from build123d import *

# Parameters (mm, degrees)
SKETCH_1_R               = 2.5
EXTRUDE_1_DEPTH          = 6
SKETCH_2_W               = 4
SKETCH_2_H               = 5
EXTRUDE_2_DEPTH          = 6
SKETCH_13_W              = 5
SKETCH_13_H              = 10
EXTRUDE_4_DEPTH          = 5
EXTRUDE_4_DEPTH_BACK     = 4.598076
SKETCH_14_W              = 5
SKETCH_14_H              = 5.9776452
CUT_EXTRUDE_6_DEPTH      = 1
CUT_EXTRUDE_6_DEPTH_BACK = 1
SKETCH_5_R               = 1
CUT_EXTRUDE_2_DEPTH      = 7
CUT_EXTRUDE_3_DEPTH      = 1.3
CUT_EXTRUDE_3_DEPTH_BACK = 1.25
SKETCH_17_W              = 2.669872981
SKETCH_17_H              = 5
CUT_EXTRUDE_8_DEPTH      = 4
FILLET_1_R               = 1
FILLET_2_R               = 3
SKETCH_15_R              = 1.5
CUT_EXTRUDE_7_DEPTH      = 5.330126966
CUT_EXTRUDE_7_DEPTH_BACK = 15.778684177
FILLET_3_R               = 1
EXTRUDE_5_DEPTH          = 1.75
SKETCH_18_W              = 6.370272001
SKETCH_18_H              = 5.288650256
CUT_EXTRUDE_9_DEPTH      = 1.5
CUT_EXTRUDE_10_DEPTH     = 1.5


with BuildPart() as part:
    # Sketch 1 → Extrude 1 (new body)
    with BuildSketch(Plane.XY):
        Circle(SKETCH_1_R)
    extrude(amount=EXTRUDE_1_DEPTH)

    # Sketch 2 → Extrude 2 (add)
    with BuildSketch(Plane(origin=(0, 0, 0), x_dir=(-1, 0, 0), z_dir=(0, 0, -1))):
        with Locations((-2, 0)):
            Rectangle(SKETCH_2_W, SKETCH_2_H)
    extrude(amount=-EXTRUDE_2_DEPTH)

    # Sketch 13 → Extrude 4 (add, two sides)
    with BuildSketch(Plane(origin=(-1.299038106, 0, 2.25), x_dir=(0, -1, 0), z_dir=(-0.5, 0, 0.866025404))) as extrude_4_sk:
        with Locations((0, 8.464101615)):
            Rectangle(SKETCH_13_W, SKETCH_13_H)
    extrude(amount=EXTRUDE_4_DEPTH)
    extrude(extrude_4_sk.sketch, amount=-EXTRUDE_4_DEPTH_BACK)

    # Sketch 14 → Cut-Extrude 6 (cut, two sides)
    with BuildSketch(Plane(origin=(-1.299038106, 0, 2.25), x_dir=(0, -1, 0), z_dir=(-0.5, 0, 0.866025404))) as cut_extrude_6_sk:
        with Locations((0, 10.475279015)):
            Rectangle(SKETCH_14_W, SKETCH_14_H)
    extrude(amount=CUT_EXTRUDE_6_DEPTH, mode=Mode.SUBTRACT)
    extrude(cut_extrude_6_sk.sketch, amount=-CUT_EXTRUDE_6_DEPTH_BACK, mode=Mode.SUBTRACT)

    # Sketch 5 → Cut-Extrude 2 (cut, through all)
    with BuildSketch(Plane.XY.offset(6)):
        with Locations((-0.639695784, 0)):
            Circle(SKETCH_5_R)
    extrude(amount=-CUT_EXTRUDE_2_DEPTH, mode=Mode.SUBTRACT)

    # Sketch 6 → Cut-Extrude 3 (cut, two sides)
    with BuildSketch(Plane.XY.offset(3)) as cut_extrude_3_sk:
        with BuildLine():
            Line((3.765698608, 2.5), (0, 2.5))
            ThreePointArc((0, 2.5), (-2.5, 0), (0, -2.5))
            Line((0, -2.5), (3.765698608, -2.5))
            Line((3.765698608, -2.5), (3.765698608, 2.5))
        make_face()
    extrude(amount=CUT_EXTRUDE_3_DEPTH, mode=Mode.SUBTRACT)
    extrude(cut_extrude_3_sk.sketch, amount=-CUT_EXTRUDE_3_DEPTH_BACK, mode=Mode.SUBTRACT)

    # Sketch 17 → Cut-Extrude 8 (cut)
    with BuildSketch(Plane(origin=(3, 0, 1.732050808), x_dir=(-0.5, 0, 0.866025404), z_dir=(-0.866025404, 0, -0.5))):
        with Locations((6.26313972, 0)):
            Rectangle(SKETCH_17_W, SKETCH_17_H)
    extrude(amount=-CUT_EXTRUDE_8_DEPTH, mode=Mode.SUBTRACT)

    # Fillet 1
    fillet_1_edges = [part.edges().sort_by_distance(p)[0] for p in [
        (2.665063509, 0, 10.312177826),
        (4, 0, 8),
    ]]
    fillet(fillet_1_edges, radius=FILLET_1_R)

    # Fillet 2
    fillet_2_edges = [part.edges().sort_by_distance(p)[0] for p in [
        (4, 0, 0),
    ]]
    fillet(fillet_2_edges, radius=FILLET_2_R)

    # Sketch 15 → Cut-Extrude 7 (cut, two sides)
    with BuildSketch(Plane(origin=(1, 0, -1.732050808), x_dir=(-0.866025404, 0, -0.5), z_dir=(0.5, 0, -0.866025404))) as cut_extrude_7_sk:
        with Locations((-10.605683392, 0)):
            Circle(SKETCH_15_R)
    extrude(amount=CUT_EXTRUDE_7_DEPTH, mode=Mode.SUBTRACT)
    extrude(cut_extrude_7_sk.sketch, amount=-CUT_EXTRUDE_7_DEPTH_BACK, mode=Mode.SUBTRACT)

    # Fillet 3
    fillet_3_edges = [part.edges().sort_by_distance(p)[0] for p in [
        (8.861215932, 2.5, 11.580127019),
        (8.861215932, -2.5, 11.580127019),
        (11.760734932, -2.5, 6.558012793),
        (11.760734932, 2.5, 6.558012793),
    ]]
    fillet(fillet_3_edges, radius=FILLET_3_R)

    # Sketch 16 → Extrude 5 (add)
    with BuildSketch(Plane(origin=(0, 0, 0), x_dir=(-1, 0, 0), z_dir=(0, 0, -1))):
        with BuildLine():
            Line((0, 2.5), (2.85, 2.5))
            Line((2.85, 2.5), (2.85, -2.5))
            Line((2.85, -2.5), (0, -2.5))
            ThreePointArc((0, -2.5), (2.5, 0), (0, 2.5))
        make_face()
    extrude(amount=-EXTRUDE_5_DEPTH)

    # Sketch 18 → Cut-Extrude 9 (cut)
    with BuildSketch(Plane(origin=(-3.799038106, 0, 6.580127019), x_dir=(0.866025404, 0, 0.5), z_dir=(-0.5, 0, 0.866025404))):
        with Locations((10.278965615, -0.144325128)):
            Rectangle(SKETCH_18_W, SKETCH_18_H)
    extrude(amount=-CUT_EXTRUDE_9_DEPTH, mode=Mode.SUBTRACT)

    # Sketch 19 → Cut-Extrude 10 (cut)
    with BuildSketch(Plane(origin=(1, 0, -1.732050808), x_dir=(-0.866025404, 0, -0.5), z_dir=(0.5, 0, -0.866025404))):
        with BuildLine():
            Line((-13.464101615, 1.5), (-13.464101615, -1.5))
            ThreePointArc((-13.464101615, -1.5), (-13.171208396, -2.207106781), (-12.464101615, -2.5))
            Line((-12.464101615, -2.5), (-7.486456415, -2.5))
            Line((-7.486456415, -2.5), (-7.486456415, 2.5))
            Line((-7.486456415, 2.5), (-12.464101615, 2.5))
            ThreePointArc((-12.464101615, 2.5), (-13.171208396, 2.207106781), (-13.464101615, 1.5))
        make_face()
    extrude(amount=-CUT_EXTRUDE_10_DEPTH, mode=Mode.SUBTRACT)


solid = part.part
For this review, take the finished solid that the model builds, in its own axes (mm). A direction names the side the tool comes from. Give positions to 0.01 mm unless a question says otherwise; leave off trailing zeros. Write each loop counter-clockwise with the first axis right and the second up, starting at its lowest first coordinate (ties: lowest second). Pieces come first, ordered by that corner, then holes. Notation, with made-up numbers: (23.25, 46.5) -> (78.25, 46.5) arc R36 ccw to (78.25, 83.5) -> close; hole circle Ø7 at (51.5, -25.75). An arc over 180 degrees is marked (long way). Use CSV: the item, a comma, the result in double quotes.
Q1. Take a section at A-A, the plane x = 2. Write out the cut boundary in (y, z).
Conclusion:
outline,"(-2.5, 0) -> (2.5, 0) -> (2.5, 1.75) -> (-2.5, 1.75) -> close; (-2.5, 4.3) -> (2.5, 4.3) -> (2.5, 6.85) -> (-2.5, 6.85) -> close"
Q2. For P1, Ø1, axis at y = -2, z = 6, coming from the +X side; P2, Ø2.5, axis at x = -0.5, y = -0.5, coming from the +Z side; P3, Ø1.8, axis at x = -0.64, y = 0, coming from the -Z side; P4, Ø1, axis at y = 0.5, z = 5.5, coming from the -X side, all flat-tipped, find the tip position at first contact; note any pin that passes through.
Conclusion:
P1,"x = 11.91"
P2,"z = 6.12"
P3,"through"
P4,"x = -2.5"
Q3. Take a section at C-C, the plane y = -0.4. State how many separate pieces and enclosed holes the cut face has, then the cut area to 3 significant figures.
Conclusion:
separate pieces,"5"
enclosed holes,"0"
area,"49.1 mm2"
Q4. Tool access review of faces 4 (the face through (7.114, -0.035, 2.652)), 5 (the face through (-2.5, 0.1, 5.1)), 6 (the face through (-2, 1, 6)): name each direction out of +Z, -Z, +X, -X, +Y, -Y from which nothing blocks a thin tool from reaching the whole face with its end or side.
Conclusion:
face 4,"+X, +Y, -Y"
face 5,"+Z, -X"
face 6,"+Z, -X, +Y, -Y"
Q5. To check wall thickness, follow probe 1 along Z at (x, y) = (-2, 0.1); probe 2 along X at (y, z) = (0.3, 5.5); probe 3 along Z at (x, y) = (1.5, 0.2). State the ranges of each line that lie inside material, in increasing order. Write a range as [from, to].
Conclusion:
probe 1,"[0, 1.75], [4.3, 6]"
probe 2,"[-2.48, -1.59], [0.31, 5.47], [6.33, 7.37]"
probe 3,"[0, 1.75], [4.3, 6.56]"
Q6. Mouldability with a two-part tool opening along Z and no side actions: class faces 1 (the face through (3.96, 0.04, 0.1)), 2 (the face through (-0.856, -0.976, 0.887)), 3 (the face through (3.766, 0, 3)) as pulls with the +Z half, pulls with the -Z half, needs draft (parallel to the pull), parting line crosses it, or undercut.
Conclusion:
face 1,"pulls with the -Z half"
face 2,"needs draft"
face 3,"undercut"
Q7. Take a section at B-B, the plane y = 1.85. Write out the cut boundary in (x, z).
Conclusion:
outline,"(-2.85, 0) -> (3.2, 0) arc R3 ccw to (4.7, 0.4) -> (7.48, 2.01) -> (6.73, 3.31) -> (11.86, 6.27) -> (10.81, 8.08) -> (5.68, 5.13) -> (4.68, 6.86) -> (9.81, 9.82) -> (8.56, 11.98) -> (3.42, 9.01) -> (3.5, 8.87) arc R1 cw to (3.13, 7.5) -> (0.54, 6) -> (-1.68, 6) -> (-1.68, 4.3) -> (3.77, 4.3) -> (3.77, 1.75) -> (-2.85, 1.75) -> close"
